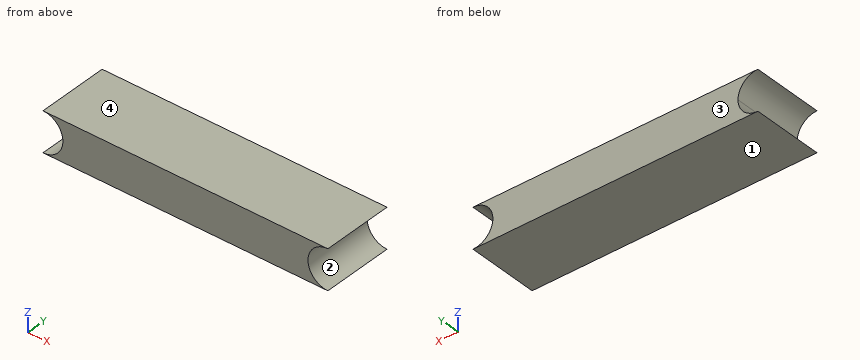
```python
from build123d import *

# Parameters (mm, degrees)
F1_DEPTH = 25


with BuildPart() as f1:
    # F0 (on Front) → F1 (new body)
    with BuildSketch(Plane.XZ):
        with BuildLine():
            ThreePointArc((6.982545, 6.982545), (4.937405, 2.04514), (0, 0))
            Line((0, 0), (100, 0))
            ThreePointArc((100, 0), (93.017455, 6.982545), (100, 13.965091))
            Line((100, 13.965091), (0, 13.965091))
            ThreePointArc((0, 13.965091), (4.937405, 11.919951), (6.982545, 6.982545))
        make_face()
    extrude(amount=F1_DEPTH)


solid = f1.part
```
Could you check a few things on this model? Use its own coordinates, in mm. Face numbers are marked on the shaded views. Round coordinates to 2 decimals unless told otherwise and drop trailing zeros. Loops run counter-clockwise (first coordinate to the right, second up) from the corner with the lowest first, then second, coordinate; pieces in that order, holes last.
Q1. I want a section at A-A (y = -3.5). Write out the boundary of the cut face in (x, z).
Q2. Thinking about a two-plate mould opening in Z: for the marked faces 1, 2, 3 and 4, which applies, pulls with the +Z half, pulls with the -Z half, needs draft (parallel to the pull), parting line crosses it, or undercut?
Q3. I want a section at B-B (z = 1). Write out the boundary of the cut face in (x, y).
Q4. Please list where these lines run through material, in increasing order: L1, parallel to Z at x = 96, y = -5.75; L2, parallel to Z at x = 96.5, y = -11.75; L3, parallel to X at y = -21.5, z = 9.25.
Q5. I want a section at C-C (z = 6). Write out the boundary of the cut face in (x, y), and give its area (3 significant figures).
Q6. For P1, Ø3, axis at y = -19.5, z = 11, coming from the -X side; P2, Ø4, axis at y = -16.5, z = 11, coming from the +X side, each with a flat end and sliding along its axis, tell me the tip position at first contact or that it passes through.
Answer below:
1. outline: (0, 0) - (100, 0) arc R6.98 cw to (100, 13.97) - (0, 13.97) arc R6.98 cw to (6.98, 6.98) arc R6.98 cw to start
2. face 1: pulls with the -Z half
2. face 2: undercut
2. face 3: needs draft
2. face 4: pulls with the +Z half
3. outline: (3.6, -25) - (96.4, -25) - (96.4, 0) - (3.6, 0) - close
4. L1: z = 0 to 1.26, 12.71 to 13.97
4. L2: z = 0 to 0.94, 13.02 to 13.97
4. L3: x = 6.6 to 93.4
5. outline: (6.91, -25) - (93.09, -25) - (93.09, 0) - (6.91, 0) - close
5. area: 2,150 mm2
6. P1: stops at x = 4.28
6. P2: stops at x = 96.46
